The figure shows three views and two pictorial views of one solid part (mm, origin at its lowest corner). Answer the questions. A direction names the side the tool comes from. Coordinates: 2 decimals unless noted, no trailing zeros. Order: outer loops, then holes, each group sorted by start corner. A loop starts at its lowest first (then second) coordinate and runs counter-clockwise, first axis right, second up. Notation, with made-up numbers: M 40,9 L 63,9 A24 ccw 63,27 Z; hole C 39,21 d5. An arc over 180 degrees is marked long. Answer in a Markdown table with one row per item. Add a question column.
Item 1: Which of the six approach directions +Z, -Z, +X, -X, +Y, -Y give full straight-line access (tool end or side, diameter ignored) to the marked faces 1 and 2?
Item 2: The part is cut by section C-C (z = 17). Write down the section's boundary in (x, y), then the cut area to 3 significant figures.
Item 3: The part is cut by section B-B (x = 45). Write down the section's boundary in (y, z).
Item 4: The part is cut by section D-D (y = 78.5). Write down the section's boundary in (x, z), then the cut area to 3 significant figures.
Item 5: Consider line 1 (X direction, y = 85, z = 43); line 2 (Y direction, x = 30, z = 30); line 3 (Z direction, x = 40, y = 105.3). Determine where each line is inside the solid, lowest interval first. Write a range as from..to.
Item 6: A flat-ended cylindrical pin translates along its axis: pin 1 Ø3 at (x, y) = (29, 81) entering from +Z. Find the tip coordinate at first contact, or state that the pin passes through.
Item 7: The part is cut by section A-A (y = 54). Write down the section's boundary in (x, z).
Item 8: The mould has two halves that part along Y. Classify the marked faces 3, 4 and 5: released by +Y, released by -Y, zero draft, split by the parting line, or undercut.
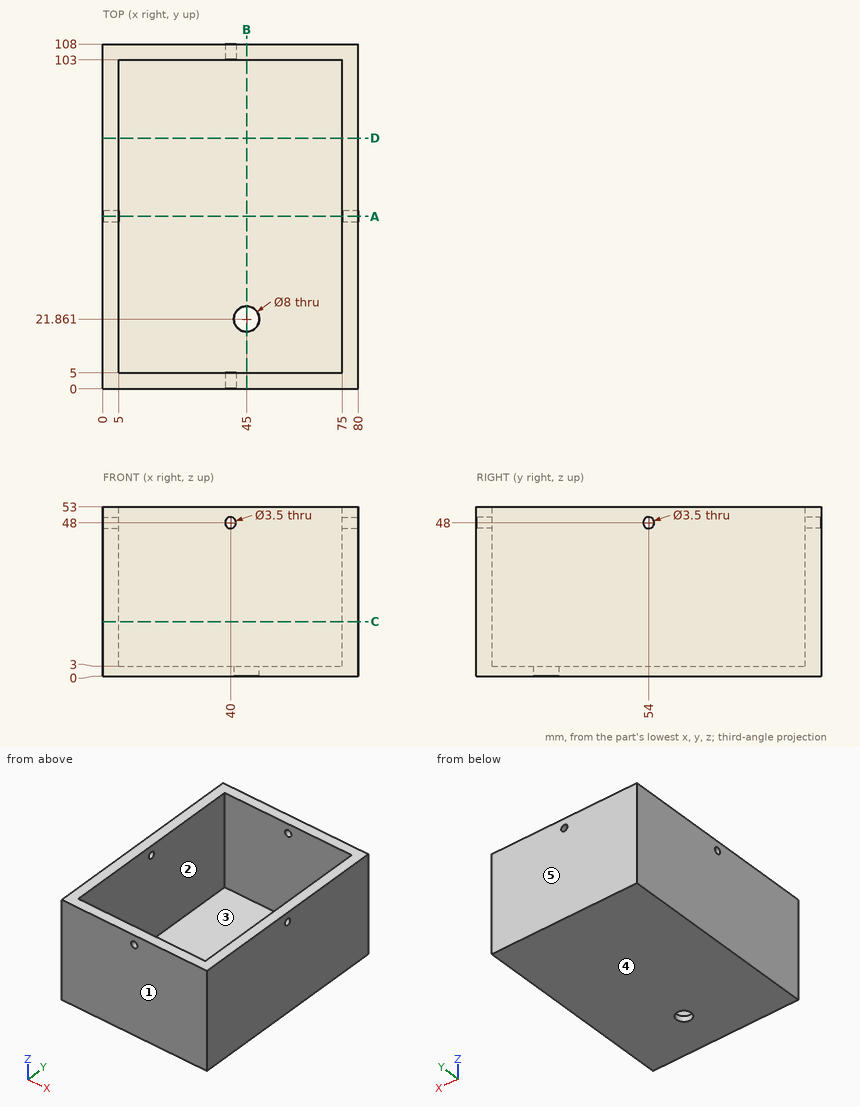
Reply:
| question | item | result |
|---|---|---|
| 1 | face 1 | +Z, -Z, +X, -X, -Y |
| 1 | face 2 | +Z |
| 2 | outline | M 0,0 L 80,0 L 80,108 L 0,108 Z; hole M 5,5 L 75,5 L 75,103 L 5,103 Z |
| 2 | area | 1,780 mm2 |
| 3 | outline | M 0,0 L 17.86,0 L 17.86,3 L 5,3 L 5,53 L 0,53 Z; M 25.86,0 L 108,0 L 108,53 L 103,53 L 103,3 L 25.86,3 Z |
| 4 | outline | M 0,0 L 80,0 L 80,53 L 75,53 L 75,3 L 5,3 L 5,53 L 0,53 Z |
| 4 | area | 740 mm2 |
| 5 | line 1 | x = 0..5, 75..80 |
| 5 | line 2 | y = 0..5, 103..108 |
| 5 | line 3 | z = 0..46.25, 49.75..53 |
| 6 | pin 1 | stops at z = 3 |
| 7 | outline | M 0,0 L 80,0 L 80,46.25 L 75,46.25 L 75,3 L 5,3 L 5,46.25 L 0,46.25 Z; M 0,49.75 L 5,49.75 L 5,53 L 0,53 Z; M 75,49.75 L 80,49.75 L 80,53 L 75,53 Z |
| 8 | face 3 | undercut |
| 8 | face 4 | zero draft |
| 8 | face 5 | released by +Y |
